CAD build for the part. Positions are in the model's coordinates, mm. Face numbers are marked on the shaded views. A direction names the side the tool comes from. Coordinates: 2 decimals unless noted, no trailing zeros. Write each loop counter-clockwise with the first axis right and the second up, starting at its lowest first coordinate (ties: lowest second). Pieces come first, ordered by that corner, then holes. Notation, with made-up numbers: (36, -19.75) -> (85, -19.75) arc R14 ccw to (85, 4.25) -> close; hole circle Ø10 at (42.5, -27). An arc over 180 degrees is marked (long way). Answer as CSV lines item,"result".
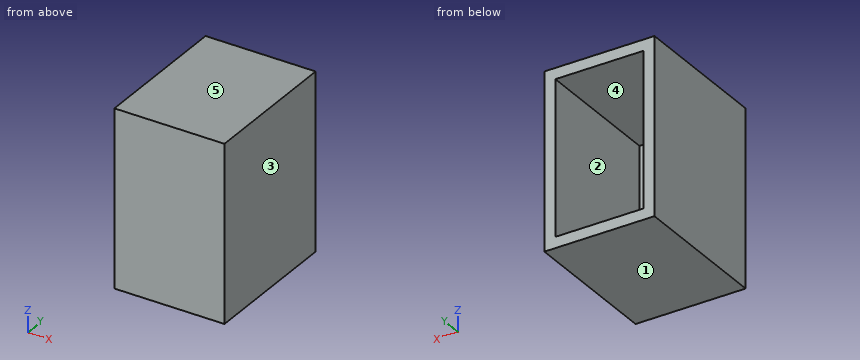
Autodesk Inventor part; units mm, degrees
ref_plane "YZ Plane" through (0, 0, 0) normal (1, 0, 0) x (0, 1, 0)
ref_plane "XZ Plane" through (0, 0, 0) normal (0, 1, 0) x (-1, 0, 0)
ref_plane "XY Plane" through (0, 0, 0) normal (0, 0, 1) x (1, 0, 0)
sketch "Boceto1" plane through (0, 0, 0) normal (0, 1, 0) x (-1, 0, 0)
  line L0 (0, 0) -> (500, 0)
  line L1 (500, 0) -> (500, -800)
  line L2 (500, -800) -> (0, -800)
  line L3 (0, -800) -> (0, 0)
  line L4 (0, 0) -> (50, 0)
  line L5 (0, -50) -> (0, 0)
  line L6 (500, -800) -> (450, -800)
  line L7 (500, -750) -> (500, -800)
  line L8 (50, -50) -> (450, -50)
  line L9 (450, -50) -> (450, -750)
  line L10 (450, -750) -> (50, -750)
  line L11 (50, -750) -> (50, -50)
  dimension "d0" = 800
  dimension "d1" = 500
  dimension "d2" = 50
  dimension "d3" = 50
extrude "Extrusión1" add sketch "Boceto1" along normal blind 600
sketch "Boceto2" plane through (0, 0, 0) normal (0, -1, 0) x (1, 0, 0)
  line L0 (0, -800) -> (-500, -800)
  line L1 (-500, -800) -> (0, -800)
  line L2 (0, -800) -> (0, 0)
  line L3 (0, 0) -> (-500, 0)
  line L4 (-500, 0) -> (-500, -800)
extrude "Extrusión2" add sketch "Boceto2" along normal blind 50
properties part number "Caja"
Item 1: Saw through at B-B on x = -345.5. Give the cut face in (y, z), and give its area (3 significant figures).
Answer below:
outline,"(-50, -800) -> (600, -800) -> (600, -750) -> (0, -750) -> (0, -50) -> (600, -50) -> (600, 0) -> (-50, 0) -> close"
area,"100,000 mm2"
Item 2: Saw through at A-A on y = 404. Give the cut face in (x, z).
Answer below:
outline,"(-500, -800) -> (0, -800) -> (0, 0) -> (-500, 0) -> close; hole (-450, -750) -> (-50, -750) -> (-50, -50) -> (-450, -50) -> close"
Item 3: 3-axis set-ups, long thin cutter, end or side, ignore diameter. For the marked faces 4 and 5: which of +Z, -Z, +X, -X, +Y, -Y reach the whole face in a straight line?
Answer below:
face 4,"+Y"
face 5,"+Z, +X, -X, +Y, -Y"
Item 4: Flat gauge pins, fed straight in: pin 1 (12 mm diameter, centred on x = -291, y = 366, fed in from +Z); pin 2 (4 mm diameter, centred on x = -297.5, z = -189, fed in from +Y). Where does each tip first touch, or does it go through?
Answer below:
pin 1,"stops at z = 0"
pin 2,"stops at y = 0"
Item 5: Saw through at C-C on z = -632. Give the cut face in (x, y), and give its area (3 significant figures).
Answer below:
outline,"(-500, -50) -> (0, -50) -> (0, 600) -> (-50, 600) -> (-50, 0) -> (-450, 0) -> (-450, 600) -> (-500, 600) -> close"
area,"85,000 mm2"
Item 6: Two-plate mould, pull along X, no slides. Class the marked faces 1, 2 and 3: pulls with the +X half, pulls with the -X half, needs draft (parallel to the pull), parting line crosses it, or undercut.
Answer below:
face 1,"needs draft"
face 2,"undercut"
face 3,"pulls with the +X half"
Item 7: Wall check: line 1 (Z direction, x = -409, y = 33.5); line 2 (X direction, y = 35.5, z = -695); line 3 (Y direction, x = -69.5, z = -120.5). Give the ranges that are in metal, low to high. Write a range as from..to.
Answer below:
line 1,"z = -800..-750, -50..0"
line 2,"x = -500..-450, -50..0"
line 3,"y = -50..0"
